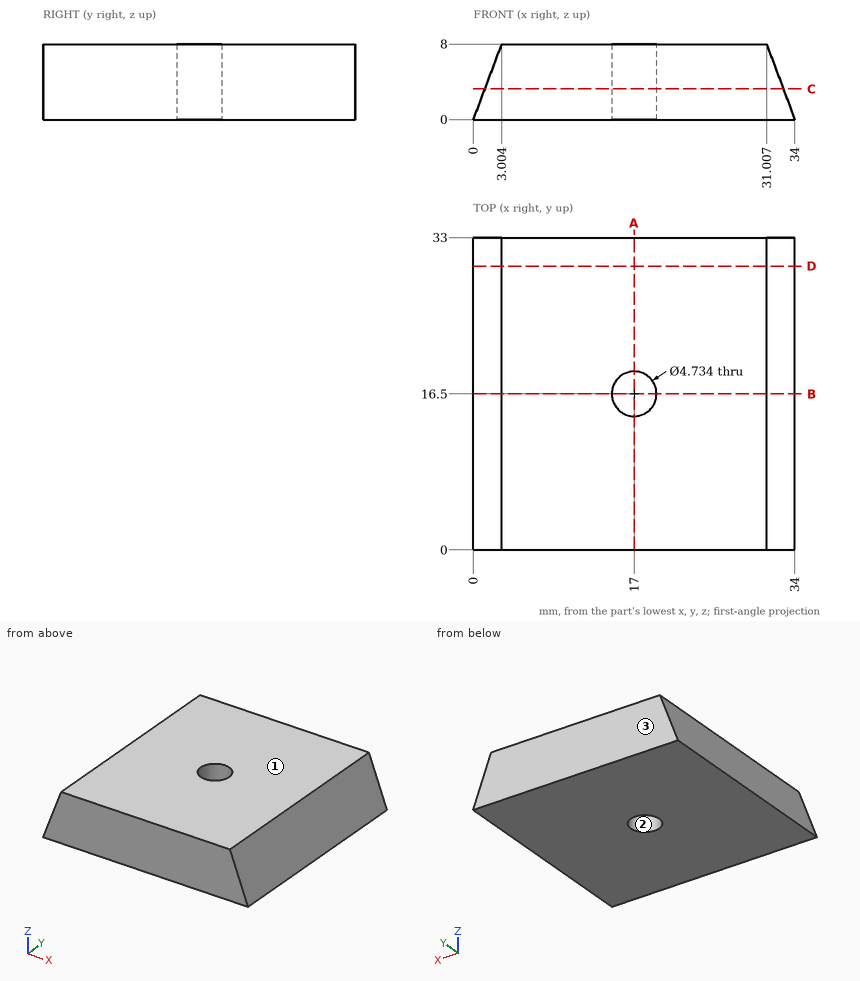
Input: dimensioned drawing with shaded views. Units: mm. Origin: part minimum x, y, z. Give positions to 0.01 mm unless a question says otherwise; leave off trailing zeros. Loops run counter-clockwise (first coordinate to the right, second up) from the corner with the lowest first, then second, coordinate; pieces in that order, holes last. Notation, with made-up numbers: M 67,30 L 96,30 A33 cw 96,59 Z; hole C -30,-4 d3. An arc over 180 degrees is marked long. Put each result on its own line as item: value.
1) Material intervals for L1, parallel to Y at x = 17, z = 6; L2, parallel to X at y = 15, z = 5; L3, parallel to Y at x = 15, z = 3.75 (1 decimal), sorted ascending. Write a range as from..to.
Computed values:
L1: y = 0..14.13, 18.87..33
L2: x = 1.88..15.17, 18.83..32.13
L3: y = 0..15.2, 17.8..33
2) Cut plane B-B, the plane y = 16.5. Return the cut outline in (x, z) (1 decimal).
Computed values:
outline: M 0,0 L 14.6,0 L 14.6,8 L 3,8 Z; M 19.4,0 L 34,0 L 31,8 L 19.4,8 Z
3) First-contact query: P1, Ø5, axis at x = 5, y = 20.5, coming from the -Z side; P2, Ø1.5, axis at y = 8.5, z = 3, coming from the -X side (1 decimal). Flat tips, straight axial feed; report the tip coordinate or a pass-through.
Computed values:
P1: stops at z = 0
P2: stops at x = 0.8
4) Mould query, pull axis Y, two halves, no side actions, for the marked faces 1, 2 and 3. Classes: released by +Y, released by -Y, zero draft, split by the parting line, or undercut.
Computed values:
face 1: zero draft
face 2: undercut
face 3: released by +Y
5) Cut plane A-A, the plane x = 17. Return the cut outline in (y, z), plus the area to 3 significant figures.
Computed values:
outline: M 0,0 L 14.13,0 L 14.13,8 L 0,8 Z; M 18.87,0 L 33,0 L 33,8 L 18.87,8 Z
area: 226 mm^2
6) Cut plane C-C, the plane z = 3.25. Return the cut outline in (x, y) (1 decimal).
Computed values:
outline: M 1.2,0 L 32.8,0 L 32.8,33 L 1.2,33 Z; hole C 17,16.5 d4.7
7) Cut plane D-D, the plane y = 30. Return the cut outline in (x, z) (1 decimal).
Computed values:
outline: M 0,0 L 34,0 L 31,8 L 3,8 Z
